The listing builds one solid part. Answer for the finished solid, in the listing's coordinates (mm). Give positions to 0.01 mm unless a question says otherwise; leave off trailing zeros. Order: outer loops, then holes, each group sorted by start corner. A loop starts at its lowest first (then second) coordinate and runs counter-clockwise, first axis right, second up.
```python
from build123d import *

# Parameters (mm, degrees)
F0_R     = 3.81
F0_R_2   = 3.175
F1_DEPTH = 6.35
F3_DEPTH = 22.86


with BuildPart() as f1:
    # F0 (on Top) → F1 (new body)
    with BuildSketch(Plane.XY):
        with Locations((0, -1.3826612849)):
            Circle(F0_R)
        with Locations((0, -1.3826612849)):
            Circle(F0_R_2, mode=Mode.SUBTRACT)
    extrude(amount=F1_DEPTH)

    # F2 (on face) → F3 (join)
    with BuildSketch(Plane.XY.offset(6.35)):
        with BuildLine():
            Line((-3.81, 2.4273387151), (-3.81, -1.3826612849))
            ThreePointArc((-3.81, -1.3826612849), (-2.6940768363, 1.3114155514), (0, 2.4273387151))
            Line((0, 2.4273387151), (-3.81, 2.4273387151))
        make_face()
        Polygon((-3.81, 2.4273387151), (0, 2.4273387151), (3.7383490708, 2.4273387151), (3.8155771326, 2.4273387151), (3.8155771326, 3.0369387151), (-3.81, 3.0369387151), align=None)
        with BuildLine():
            Line((3.7383490708, 2.4273387151), (0, 2.4273387151))
            ThreePointArc((0, 2.4273387151), (2.6429446594, 1.3615951767), (3.8073060154, -1.2394100895))
            Line((3.8073060154, -1.2394100895), (3.7383490708, 2.4273387151))
        make_face()
    extrude(amount=-F3_DEPTH)


solid = f1.part
```
1) Given P1, Ø1, axis at y = -1.5, z = 3, coming from the +X side; P2, Ø1, axis at x = 3, y = -4, coming from the -Z side, each flat-ended and moving along its own axis, determine where each tip first touches the part or whether it passes through.
Geometry says:
P1: stops at x = 3.81
P2: stops at z = 0
2) Find section A-A (y = -2). Write down the section's boundary in (x, z), then the cut area to 3 significant figures.
Geometry says:
outline: (-3.76, 0) - (-3.11, 0) - (-3.11, 6.35) - (-3.76, 6.35) - close; (3.11, 0) - (3.76, 0) - (3.76, 6.35) - (3.11, 6.35) - close
area: 8.19 mm2
3) For a pull along X with two mould halves and no side action, classify faces 1 (the cylindrical face through (-0.013, -5.193, 3.131)), 2 (the flat face through (-1, 2, 0)), 3 (the flat face through (0, 2.6, -16.51)) as +X half, -X half, draft (parallel to the pull), parting line (faces both ways), or undercut.
Geometry says:
face 1: parting line
face 2: undercut
face 3: draft
4) Straight lines are drawn through the part: probe 1 along Y at (x, z) = (0, 4.5); probe 2 along X at (y, z) = (-1, 4.25); probe 3 along Z at (x, y) = (-3, 0.5). For each, find the intervals that lie inside material, in ascending order.
Geometry says:
probe 1: y = -5.19 to -4.56, 1.79 to 3.04
probe 2: x = -3.81 to -3.15, 3.15 to 3.8
probe 3: z = 0 to 6.35
5) Find section C-C (x = -2). Write down the section's boundary in (y, z).
Geometry says:
outline: (-4.63, 0) - (-3.85, 0) - (-3.85, 6.35) - (-4.63, 6.35) - close; (1.08, 0) - (1.86, 0) - (1.86, -16.51) - (3.04, -16.51) - (3.04, 6.35) - (1.08, 6.35) - close
6) Find section D-D (y = 2). Write down the section's boundary in (x, z).
Geometry says:
outline: (-3.81, -16.51) - (-1.75, -16.51) - (-1.75, 0) - (1.75, 0) - (1.75, -16.51) - (3.75, -16.51) - (3.75, 6.35) - (-3.81, 6.35) - close
